Build history of the part. All positions in model axes, mm. Round coordinates to 2 decimals unless told otherwise and drop trailing zeros. Write each loop counter-clockwise with the first axis right and the second up, starting at its lowest first coordinate (ties: lowest second). Pieces come first, ordered by that corner, then holes. Notation, with made-up numbers: M 79.25,29.5 L 122.25,29.5 A12 ccw 122.25,33.5 Z; hole C 11,-33.75 d3. An arc over 180 degrees is marked long. Use a Markdown table: item, result.
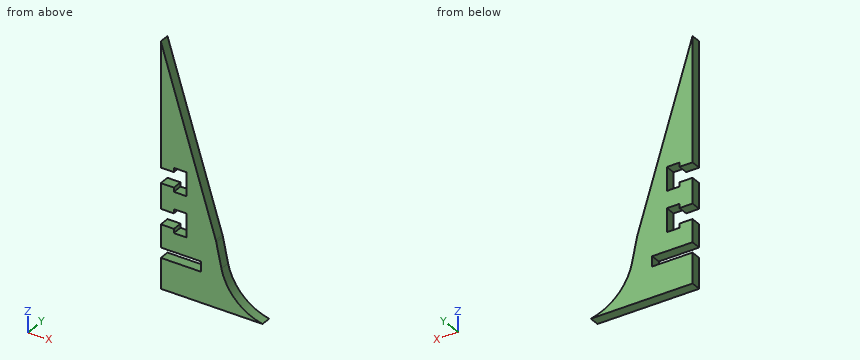
from build123d import *

# Parameters (mm, degrees)
F1_DEPTH = 3.175


with BuildPart() as f1:
    # F0 (on Front) → F1 (new body)
    with BuildSketch(Plane.XZ):
        with BuildLine():
            ThreePointArc((19.272455, -76.2), (10.907118, -71.787462), (6.35, -63.5))
            Line((6.35, -63.5), (4.726481, -55.935776))
            ThreePointArc((4.726481, -55.935776), (4.659413, -55.65464), (4.579622, -55.376848))
            Line((4.579622, -55.376848), (-12.7, 0))
            Line((-12.7, 0), (-12.7, -38.89375))
            Line((-12.7, -38.89375), (-8.587963, -38.89375))
            Line((-8.587963, -38.89375), (-8.587963, -37.58333))
            Line((-8.587963, -37.58333), (-4.619213, -37.58333))
            Line((-4.619213, -37.58333), (-4.619213, -44.96667))
            Line((-4.619213, -44.96667), (-8.587963, -44.96667))
            Line((-8.587963, -44.96667), (-8.587963, -43.65625))
            Line((-8.587963, -43.65625), (-12.7, -43.65625))
            Line((-12.7, -43.65625), (-12.7, -51.59375))
            Line((-12.7, -51.59375), (-8.587963, -51.59375))
            Line((-8.587963, -51.59375), (-8.587963, -50.28333))
            Line((-8.587963, -50.28333), (-4.619213, -50.28333))
            Line((-4.619213, -50.28333), (-4.619213, -57.66667))
            Line((-4.619213, -57.66667), (-8.587963, -57.66667))
            Line((-8.587963, -57.66667), (-8.587963, -56.35625))
            Line((-8.587963, -56.35625), (-12.7, -56.35625))
            Line((-12.7, -56.35625), (-12.7, -63.5))
            Line((-12.7, -63.5), (0, -63.5))
            Line((0, -63.5), (0, -66.675))
            Line((0, -66.675), (-12.7, -66.675))
            Line((-12.7, -66.675), (-12.7, -76.2))
            Line((-12.7, -76.2), (19.272455, -76.2))
        make_face()
    extrude(amount=F1_DEPTH)


solid = f1.part
Q1. Cut at C-C on z = -8. Give the cut face in (x, y) (3 decimals).
Response values:
| item | result |
|---|---|
| outline | M -12.7,-3.175 L -10.204,-3.175 L -10.204,0 L -12.7,0 Z |
Q2. Drill centre lines: L1, parallel to X at y = -0.6, z = -38.5; L2, parallel to X at y = -0.95, z = -15; L3, parallel to Z at x = 11, y = -3. Where is each one in solid material? Low to high.
Response values:
| item | result |
|---|---|
| L1 | x = -12.7 to -8.59, -4.62 to -0.69 |
| L2 | x = -12.7 to -8.02 |
| L3 | z = -76.2 to -71.88 |
Q3. Cut at A-A on y = -1.5. Give the cut face in (x, z) (3 decimals).
Response values:
| item | result |
|---|---|
| outline | M -12.7,-76.2 L 19.272,-76.2 A16.464 cw 6.35,-63.5 L 4.726,-55.936 A6.35 ccw 4.58,-55.377 L -12.7,0 L -12.7,-38.894 L -8.588,-38.894 L -8.588,-37.583 L -4.619,-37.583 L -4.619,-44.967 L -8.588,-44.967 L -8.588,-43.656 L -12.7,-43.656 L -12.7,-51.594 L -8.588,-51.594 L -8.588,-50.283 L -4.619,-50.283 L -4.619,-57.667 L -8.588,-57.667 L -8.588,-56.356 L -12.7,-56.356 L -12.7,-63.5 L 0,-63.5 L 0,-66.675 L -12.7,-66.675 Z |
Q4. Cut at B-B on x = -3. Give the cut face in (y, z) (3 decimals).
Response values:
| item | result |
|---|---|
| outline | M -3.175,-76.2 L 0,-76.2 L 0,-66.675 L -3.175,-66.675 Z; M -3.175,-63.5 L 0,-63.5 L 0,-31.086 L -3.175,-31.086 Z |
Q5. Drop flat-ended pins along their axis: P1, Ø1, axis at y = -2.5, z = -60, coming from the +X side; P2, Ø0.7, axis at y = -1.5, z = -44, coming from the +X side; P3, Ø1.4, axis at y = -1, z = -38, coming from the +X side. Give the stop position or say it passes through.
Response values:
| item | result |
|---|---|
| P1 | stops at x = 5.71 |
| P2 | stops at x = 1.14 |
| P3 | stops at x = -0.62 |
Q6. Cut at D-D on x = 11.5. Give the cut face in (y, z) (3 decimals).
Response values:
| item | result |
|---|---|
| outline | M -3.175,-76.2 L 0,-76.2 L 0,-72.342 L -3.175,-72.342 Z |
